Build history of the part. All positions in model axes, mm. A direction names the side the tool comes from. Give positions to 0.01 mm unless a question says otherwise; leave off trailing zeros. Order: outer loops, then holes, each group sorted by start corner. A loop starts at its lowest first (then second) coordinate and runs counter-clockwise, first axis right, second up. Notation, with made-up numbers: M -39,47.5 L 4,47.5 A26 ccw 4,75.5 Z; hole C -34.5,44.5 d8. An arc over 180 degrees is marked long. One line per item, written item: value.
from build123d import *

# Parameters (mm, degrees)
SKETCH_1_R          = 0.6
EXTRUDE_1_DEPTH     = 30
SKETCH_2_R          = 1.837847415
EXTRUDE_2_DEPTH     = 1
SKETCH_3_R          = 0.665703361
CUT_EXTRUDE_1_DEPTH = 32.999712653


with BuildPart() as part:
    # 草图1 → 凸台-拉伸1 (new body)
    with BuildSketch(Plane(origin=(0, 0, 0), x_dir=(0, 0, -1), z_dir=(1, 0, 0))):
        Circle(SKETCH_1_R)
    extrude(amount=EXTRUDE_1_DEPTH)

    # 草图2 → 凸台-拉伸2 (add, symmetric)
    with BuildSketch(Plane(origin=(8.379426917, -0.245734266, -12), x_dir=(1, 0, 0), z_dir=(0, 1, 0))):
        with Locations(Location((21.666952485, -12, 0), (0, 0, 270))):
            Circle(SKETCH_2_R)
    extrude(amount=EXTRUDE_2_DEPTH, both=True)

    # 草图3 → 切除-拉伸1 (cut, through all)
    with BuildSketch(Plane(origin=(0, -1.245734266, 0), x_dir=(-1, 0, 0), z_dir=(0, -1, 0))):
        with Locations(Location((-30.046379401, 0, 0), (0, 0, 90))):
            Circle(SKETCH_3_R)
    extrude(amount=-CUT_EXTRUDE_1_DEPTH, mode=Mode.SUBTRACT)


solid = part.part
1) Tool access for faces 5 (the face through (30, 0.754, 1)), 6 (the face through (13.956, 0.506, -0.323)): list every direction of +Z, -Z, +X, -X, +Y, -Y with a clear straight run to the whole face (end or side of a thin tool).
Check values:
face 5: +Z, -Z, +X, -X, +Y
face 6: -X
2) Drill centre lines: probe 1 along X at (y, z) = (0.25, 0); probe 2 along X at (y, z) = (-0.75, 0); probe 3 along Z at (x, y) = (5.5, 0.05). Where is each one in solid material? Low to high. Write a range as from..to.
Check values:
probe 1: 0..29.38, 30.71..31.88
probe 2: 28.21..29.38, 30.71..31.88
probe 3: -0.6..0.6
3) Mould opens along X. For faces 1 (the face through (31.87, -0.23, -0.24)), 2 (the face through (0, 0, 0)), 3 (the face through (30.706, -0.26, 0.087)), 4 (the face through (30, -1.246, 1)) say: released by +X, released by -X, zero draft, split by the parting line, or undercut.
Check values:
face 1: split by the parting line
face 2: released by -X
face 3: undercut
face 4: zero draft
4) Saw through at A-A, the plane z = 0. Write the cut outline in (x, y).
Check values:
outline: M 0,-0.6 L 28.21,-0.6 L 28.21,-1.25 L 29.38,-1.25 L 29.38,0.75 L 28.21,0.75 L 28.21,0.6 L 0,0.6 Z; M 30.71,-1.25 L 31.88,-1.25 L 31.88,0.75 L 30.71,0.75 Z
5) Saw through at C-C, the plane x = 17. Write the cut outline in (y, z), then the cut area to 3 significant figures.
Check values:
outline: C 0,0 d1.2
area: 1.13 mm^2
6) Pin check, flat tip, straight feed: pin 1 (1 mm diameter, centred on x = 26, y = 0.5, fed in from +Z). Stop position of the tip, or through.
Check values:
pin 1: z = 0.6
7) Saw through at B-B, the plane y = 0. Write the cut outline in (x, z).
Check values:
outline: M 0,-0.6 L 28.31,-0.6 A1.84 ccw long 28.31,0.6 L 0,0.6 Z; hole C 30.05,0 d1.33
